Check sheet for the drawn part. Datum: minimum x, y, z corner. Units: mm. A direction names the side the tool comes from. Coordinates: 2 decimals unless noted, no trailing zeros. Order: outer loops, then holes, each group sorted by start corner. A loop starts at its lowest first (then second) coordinate and runs counter-clockwise, first axis right, second up. Notation, with made-up numbers: (-13, 65.25) - (3, 65.25) arc R19 cw to (3, 95.25) - close; hole circle Ø3 at (55, -16.5). An arc over 180 degrees is marked (long way). Answer as CSV lines item,"result". Start each with the question number.
1. Section check C-C (z = 52.5). Record the cut outline in (x, y), and give its area (3 significant figures).
2. Section check B-B (y = 35). Record the cut outline in (x, z), and give its area (3 significant figures).
3. Section check A-A (x = 426.5). Record the cut outline in (y, z), and give its area (3 significant figures).
4. Section check D-D (y = 92). Record the cut outline in (x, z), and give its area (3 significant figures).
5. Mould release check, pull along X, two halves, no side actions. Record for the marked faces 4, 5 and 6: pulls with the +X half, pulls with the -X half, needs draft (parallel to the pull), parting line crosses it, or undercut.
6. Material ranges on L1, parallel to Z at x = 435.5, y = 11.5; L2, parallel to X at y = 37, z = 54.5; L3, parallel to Z at x = 177.5, y = 101.5, recorded low to high. Write a range as [from, to].
7. Go/stop test with flat-tipped pins: pin 1 (1.5 mm diameter, centred on x = 440.5, z = 34, fed in from -Y); pin 2 (4 mm diameter, centred on y = 88.5, z = 208, fed in from +X); pin 3 (3 mm diameter, centred on x = 327.5, y = 16.5, fed in from +Z). Record where each tip stops, or that it passes through.
8. Set-up check for the marked faces 1, 2 and 3: record each of +Z, -Z, +X, -X, +Y, -Y from which the full face is reachable in a straight line by a thin tool's end or side.
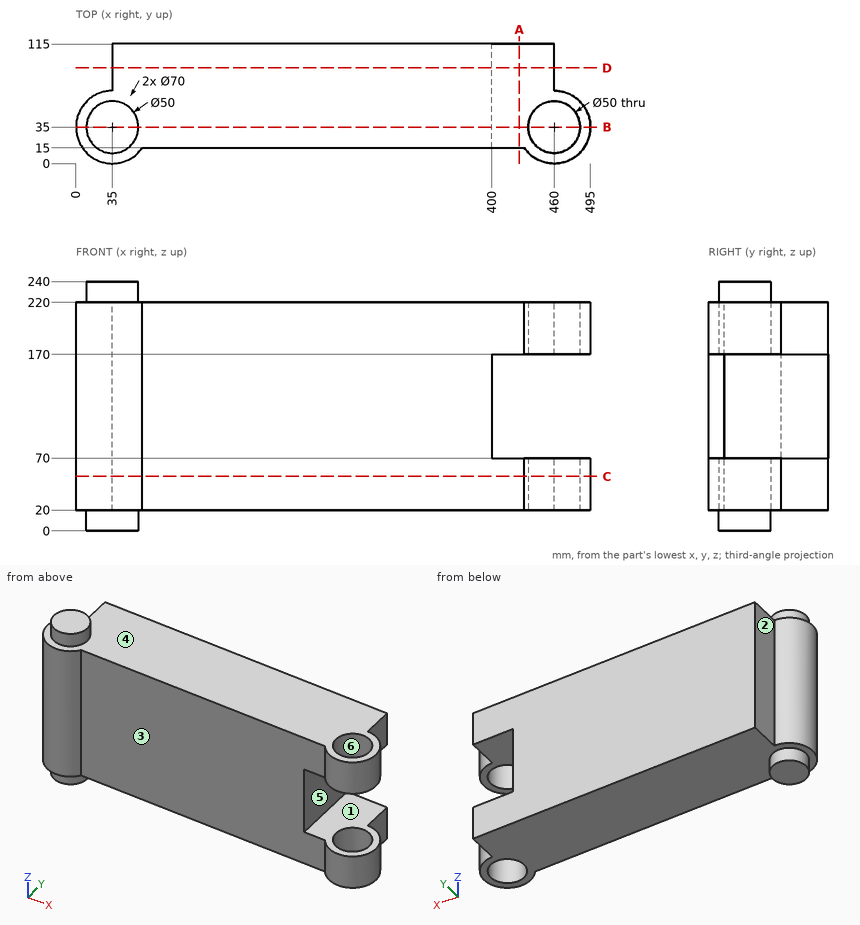
Evaluation:
1,outline,"(35, 70) arc R35 ccw (long way) to (63.72, 15) - (431.28, 15) arc R35 ccw (long way) to (460, 70) - (460, 115) - (35, 115) - close; hole circle Ø50 at (460, 35)"
1,area,"45,000 mm²"
2,outline,"(0, 20) - (10, 20) - (10, 0) - (60, 0) - (60, 20) - (435, 20) - (435, 70) - (400, 70) - (400, 170) - (435, 170) - (435, 220) - (60, 220) - (60, 240) - (10, 240) - (10, 220) - (0, 220) - close; (485, 20) - (495, 20) - (495, 70) - (485, 70) - close; (485, 170) - (495, 170) - (495, 220) - (485, 220) - close"
2,area,"86,500 mm²"
3,outline,"(15, 20) - (115, 20) - (115, 70) - (15, 70) - close; (15, 170) - (115, 170) - (115, 220) - (15, 220) - close"
3,area,"10,000 mm²"
4,outline,"(35, 20) - (460, 20) - (460, 70) - (400, 70) - (400, 170) - (460, 170) - (460, 220) - (35, 220) - close"
4,area,"79,000 mm²"
5,face 4,"needs draft"
5,face 5,"pulls with the +X half"
5,face 6,"undercut"
6,L1,"z = [20, 70], [170, 220]"
6,L2,"x = [0.06, 435.08], [484.92, 494.94]"
6,L3,"z = [20, 220]"
7,pin 1,"stops at y = 5.45"
7,pin 2,"stops at x = 460"
7,pin 3,"stops at z = 220"
8,face 1,"+X, +Y, -Y"
8,face 2,"+Z, -Z, -X, +Y"
8,face 3,"+Z, -Z, -Y"
